from build123d import *

# Parameters (mm, degrees)
F1_DEPTH = 3


with BuildPart() as f1:
    # F0 (on Top) → F1 (new body)
    with BuildSketch(Plane.XY):
        with BuildLine():
            ThreePointArc((-39.498382, 0), (-36.379069, 7.530687), (-28.848382, 10.65))
            Line((-28.848382, 10.65), (-39.498382, 10.65))
            Line((-39.498382, 10.65), (-39.498382, 0))
        make_face()
        with BuildLine():
            Line((-17.65, 10.65), (-28.848382, 10.65))
            ThreePointArc((-28.848382, 10.65), (-36.379069, 7.530687), (-39.498382, 0))
            ThreePointArc((-39.498382, 0), (-36.379069, -7.530687), (-28.848382, -10.65))
            Line((-28.848382, -10.65), (-17.65, -10.65))
            ThreePointArc((-17.65, -10.65), (-10.119313, -7.530687), (-7, 0))
            ThreePointArc((-7, 0), (-7.158698, 1.831689), (-7.630063, 3.608788))
            ThreePointArc((-7.630063, 3.608788), (-11.526729, 8.71367), (-17.65, 10.65))
        make_face()
        with BuildLine():
            ThreePointArc((-17.65, 7.65), (-10, 0), (-17.65, -7.65))
            Line((-17.65, -7.65), (-28.848382, -7.65))
            ThreePointArc((-28.848382, -7.65), (-36.498382, 0), (-28.848382, 7.65))
            Line((-28.848382, 7.65), (-17.65, 7.65))
        make_face(mode=Mode.SUBTRACT)
        with BuildLine():
            ThreePointArc((7.630063, 3.608788), (0, 6.350694), (-7.630063, 3.608788))
            ThreePointArc((-7.630063, 3.608788), (-7.158698, 1.831689), (-7, 0))
            ThreePointArc((-7, 0), (0, 3.350694), (7, 0))
            ThreePointArc((7, 0), (7.158698, 1.831689), (7.630063, 3.608788))
        make_face()
        with BuildLine():
            ThreePointArc((17.65, 10.65), (11.526729, 8.71367), (7.630063, 3.608788))
            ThreePointArc((7.630063, 3.608788), (7.158698, 1.831689), (7, 0))
            ThreePointArc((7, 0), (10.119313, -7.530687), (17.65, -10.65))
            Line((17.65, -10.65), (28.848382, -10.65))
            ThreePointArc((28.848382, -10.65), (36.379069, -7.530687), (39.498382, 0))
            ThreePointArc((39.498382, 0), (36.379069, 7.530687), (28.848382, 10.65))
            Line((28.848382, 10.65), (17.65, 10.65))
        make_face()
        with BuildLine():
            Line((28.848382, -7.65), (17.65, -7.65))
            ThreePointArc((17.65, -7.65), (10, 0), (17.65, 7.65))
            Line((17.65, 7.65), (28.848382, 7.65))
            ThreePointArc((28.848382, 7.65), (36.498382, 0), (28.848382, -7.65))
        make_face(mode=Mode.SUBTRACT)
        with BuildLine():
            Line((39.498382, 10.65), (28.848382, 10.65))
            ThreePointArc((28.848382, 10.65), (36.379069, 7.530687), (39.498382, 0))
            Line((39.498382, 0), (39.498382, 10.65))
        make_face()
    extrude(amount=F1_DEPTH)


solid = f1.part
Design review of the part built by this model. Coordinates are the model's own, in mm. A direction names the side the tool comes from. Give positions to 0.01 mm unless a question says otherwise; leave off trailing zeros. Loops run counter-clockwise (first coordinate to the right, second up) from the corner with the lowest first, then second, coordinate; pieces in that order, holes last. Notation, with made-up numbers: M 31.5,-1.5 L 90.5,-1.5 A24 ccw 90.5,16.5 Z; hole C 82.25,88.5 d11. An arc over 180 degrees is marked long. Write item = value, one per line.
Q1. To check wall thickness, follow line 1 (X direction, y = -3.75, z = 2.25); line 2 (X direction, y = -6.5, z = 2.35); line 3 (Y direction, x = 24.5, z = 1.1). State the ranges of each line that lie inside material, in increasing order. Write a range as [from, to].
Output values:
line_1 = [-38.82, -35.52], [-10.98, -7.68], [7.68, 10.98], [35.52, 38.82]
line_2 = [-37.28, -32.88], [-13.62, -9.21], [9.21, 13.62], [32.88, 37.28]
line_3 = [-10.65, -7.65], [7.65, 10.65]
Q2. We need section A-A (z = 2.15). Give the boundary of the cut face in (x, y), plus the area to 3 significant figures.
Output values:
outline = M -39.5,0 A10.65 ccw -28.85,-10.65 L -17.65,-10.65 A10.65 ccw -7,0 A8.99 cw 7,0 A10.65 ccw 17.65,-10.65 L 28.85,-10.65 A10.65 ccw 39.5,0 L 39.5,10.65 L 17.65,10.65 A10.65 ccw 7.63,3.61 A11.99 ccw -7.63,3.61 A10.65 ccw -17.65,10.65 L -39.5,10.65 Z; hole M -28.85,-7.65 L -17.65,-7.65 A7.65 ccw -17.65,7.65 L -28.85,7.65 A7.65 ccw Z; hole M 17.65,-7.65 L 28.85,-7.65 A7.65 ccw 28.85,7.65 L 17.65,7.65 A7.65 ccw Z
area = 576 mm^2
Q3. We need section C-C (x = 12). Give the boundary of the cut face in (y, z), plus the area to 3 significant figures.
Output values:
outline = M -9.03,0 L -5.16,0 L -5.16,3 L -9.03,3 Z; M 5.16,0 L 9.03,0 L 9.03,3 L 5.16,3 Z
area = 23.2 mm^2
Q4. Draft analysis for pull direction Y (two halves, no side actions). For faces 1 (the flat face through (0, 5, 0)), 2 (the cylindrical face through (36.3, -7.61, 1.48)), 3 (the cylindrical face through (10, 0, 1)), state which applies: +Y half, -Y half, draft (parallel to the pull), parting line (faces both ways), or undercut.
Output values:
face_1 = draft
face_2 = -Y half
face_3 = undercut
Q5. We need section B-B (y = 0.75). Give the boundary of the cut face in (x, z).
Output values:
outline = M -39.5,0 L -36.46,0 L -36.46,3 L -39.5,3 Z; M -10.04,0 L -6.32,0 L -6.32,3 L -10.04,3 Z; M 6.32,0 L 10.04,0 L 10.04,3 L 6.32,3 Z; M 36.46,0 L 39.5,0 L 39.5,3 L 36.46,3 Z
Q6. For faces 4 (the flat face through (-23, -7.65, 1)), 5 (the flat face through (-23, -10.65, 1)), 6 (the cylindrical face through (10.04, -7.45, 1.48)), list the 3-axis set-ups (+Z, -Z, +X, -X, +Y, -Y) from which the entire face can be reached by the end or side of a thin tool; tool diameter is ignored.
Output values:
face_4 = +Z, -Z
face_5 = +Z, -Z, +X, -X, -Y
face_6 = +Z, -Z, -Y
Q7. We need section D-D (y = 4.75). Give the boundary of the cut face in (x, z), plus the area to 3 significant figures.
Output values:
outline = M -39.5,0 L -34.85,0 L -34.85,3 L -39.5,3 Z; M -11.65,0 L -8.12,0 L -8.12,3 L -11.65,3 Z; M -5.98,0 L 5.98,0 L 5.98,3 L -5.98,3 Z; M 8.12,0 L 11.65,0 L 11.65,3 L 8.12,3 Z; M 34.85,0 L 39.5,0 L 39.5,3 L 34.85,3 Z
area = 85.0 mm^2
